Verification items for this drawing (mm, ordinates from the low corner). A direction names the side the tool comes from. Coordinates: 2 decimals unless noted, no trailing zeros. Write each loop counter-clockwise with the first axis right and the second up, starting at its lowest first coordinate (ties: lowest second). Pieces come first, ordered by that corner, then holes. Notation, with made-up numbers: (-29.5, 61) -> (24.5, 61) arc R23 cw to (24.5, 69) -> close; hole circle Ø1 at (87, 21). An arc over 180 degrees is marked (long way). One line per item, written item: value. Start each with the question number.
1) Set-up check for the marked faces 1, 2 and 3: record each of +Z, -Z, +X, -X, +Y, -Y from which the full face is reachable in a straight line by a thin tool's end or side.
2) Sectioned sample at B-B on z = 2.5. Give the number of separate pieces and of enclosed holes in the cut face, plus the area to 3 significant figures.
3) Scan lines: line 1 along X through (y, z) = (0.8, 3.1); line 2 along X through (y, z) = (0.25, 3.25); line 3 along X through (y, z) = (2.95, 3.55). Record each from-to range of solid material in increasing order. Write a range as [from, to].
4) Sectioned sample at A-A on x = 43. Enter the section's corners in (y, z), plus the area to 3 significant figures.
5) Gauge pin test, flat ends, axial feed: P1, Ø2, axis at y = 3.5, z = 3, coming from the -X side; P2, Ø2.5, axis at x = 5, z = 3.5, coming from the +Y side; P3, Ø0.5, axis at y = 2.5, z = 2, coming from the +X side; P4, Ø3, axis at x = 28, y = 2, coming from the -Z side. Record the tip position at first contact, or that the pin passes through.
6) Sectioned sample at C-C on x = 5. Enter the section's corners in (y, z), plus the area to 3 significant figures.
7) Sectioned sample at D-D on x = 19. Enter the section's corners in (y, z), plus the area to 3 significant figures.
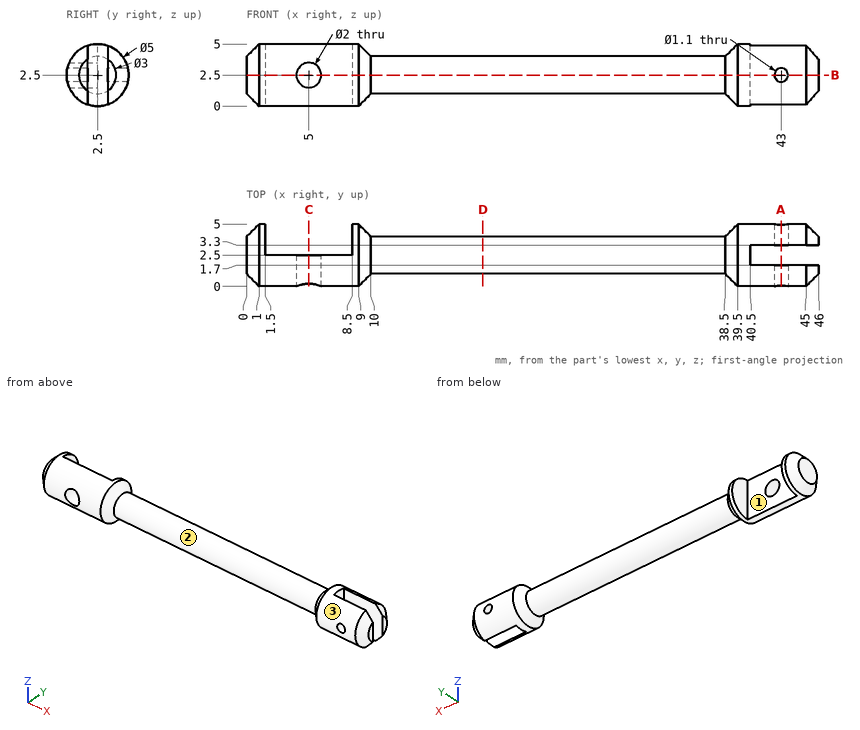
Answers:
1. face 1: +Z, -Z, +Y
1. face 2: none
1. face 3: +X, -X
2. separate pieces: 4
2. enclosed holes: 0
2. area: 134 mm2
3. line 1: x = [0.3, 4.2], [5.8, 9.7], [38.8, 45.7]
3. line 2: x = [0.87, 4.34], [5.66, 9.13], [39.37, 45.13]
3. line 3: x = [0, 1.5], [8.5, 40.5]
4. outline: (0.06, 1.95) arc R2.5 ccw to (1.7, 0.13) -> (1.7, 1.95) -> close; (0.06, 3.05) -> (1.7, 3.05) -> (1.7, 4.87) arc R2.5 ccw to start; (3.3, 0.13) arc R2.5 ccw to (4.94, 1.95) -> (3.3, 1.95) -> close; (3.3, 3.05) -> (4.94, 3.05) arc R2.5 ccw to (3.3, 4.87) -> close
4. area: 8.08 mm2
5. P1: stops at x = 0
5. P2: stops at y = 2.5
5. P3: stops at x = 40.5
5. P4: stops at z = 1
6. outline: (0.21, 1.5) arc R2.5 ccw to (2.5, 0) -> (2.5, 1.5) -> close; (0.21, 3.5) -> (2.5, 3.5) -> (2.5, 5) arc R2.5 ccw to start
6. area: 4.95 mm2
7. outline: circle Ø3 at (2.5, 2.5)
7. area: 7.07 mm2
